Read the model definition and answer for the solid it produces. Units are mm, in the model's axes. Give positions to 0.01 mm unless a question says otherwise; leave off trailing zeros. Order: outer loops, then holes, each group sorted by start corner. A loop starts at its lowest first (then second) coordinate and runs counter-clockwise, first axis right, second up. Notation, with made-up numbers: (-25, 0.5) - (-8, 0.5) arc R27 ccw to (-8, 34.5) - close; hole circle Ø4 at (77, 1.25). An arc over 180 degrees is marked (long way). Write each question's results on one line, items separated by ' | '. Start each with the question number.
Q1. For a pull along Y with two mould halves and no side action, classify faces 1 (the face through (8, 0, 5)), 2 (the face through (14, 50.8, 5)), 3 (the face through (15.994, 28.43, 5.009)), 4 (the face through (16.365, 1.81, 5.151)) as +Y half, -Y half, draft (parallel to the pull), parting line (faces both ways), or undercut.
Q2. Find section D-D on y = 9. Give the vertices of the cut face in (x, z), and give its area (3 significant figures).
Q3. Find section A-A on z = 3.75. Give the vertices of the cut face in (x, y) (3 decimals).
Q4. Find section C-C on x = 3. Give the vertices of the cut face in (y, z).
Q5. Find section B-B on y = 2.54. Give the vertices of the cut face in (x, z), and give its area (3 significant figures).
Q6. Flat-ended cylindrical pins translate along their axes: P1, Ø3, axis at x = 4.5, z = 6, coming from the +Y side; P2, Ø2, axis at y = 44, z = 7.5, coming from the +X side. Find the tip coordinate at first contact, or state that the pin passes through.
Q7. Find the intervals of material crossed by line 1 along Y through (x, z) = (5.5, 1.25); line 2 along X through (y, z) = (26, 6); line 3 along X through (y, z) = (42.5, 1.25), in increasing order. Write a range as from..to.
from build123d import *

# Parameters (mm, degrees)
BOSS_EXTRUDE1_DEPTH     = 10.16
SKETCH2_R               = 1.905
CUT_EXTRUDE1_DEPTH      = 1
CUT_EXTRUDE1_DEPTH_BACK = 11.16


with BuildPart() as part:
    # Sketch1 → Boss-Extrude1 (new body)
    with BuildSketch(Plane.XY):
        with BuildLine():
            Line((0, 0), (16.51, 0))
            ThreePointArc((16.51, 0), (21.143005914, 25.4), (16.51, 50.8))
            Line((16.51, 50.8), (11.050639123, 50.8))
            ThreePointArc((11.050639123, 50.8), (16.008340976, 28.103171462), (12.900542854, 5.08))
            Line((12.900542854, 5.08), (0, 5.08))
            Line((0, 5.08), (0, 0))
        make_face()
    extrude(amount=BOSS_EXTRUDE1_DEPTH)

    # Sketch2 → Cut-Extrude1 (cut, two sides)
    with BuildSketch(Plane.XY.offset(10.16)) as cut_extrude1_sk:
        with Locations((14.605, 2.54)):
            Circle(SKETCH2_R)
    extrude(amount=CUT_EXTRUDE1_DEPTH, mode=Mode.SUBTRACT)
    extrude(cut_extrude1_sk.sketch, amount=-CUT_EXTRUDE1_DEPTH_BACK, mode=Mode.SUBTRACT)


solid = part.part
Working result:
1) face 1: -Y half | face 2: +Y half | face 3: undercut | face 4: undercut
2) outline: (14.02, 0) - (19.25, 0) - (19.25, 10.16) - (14.02, 10.16) - close | area: 53.1 mm²
3) outline: (0, 0) - (16.51, 0) arc R71.943 ccw to (16.51, 50.8) - (11.051, 50.8) arc R66.863 cw to (12.901, 5.08) - (0, 5.08) - close; hole circle Ø3.81 at (14.605, 2.54)
4) outline: (0, 0) - (5.08, 0) - (5.08, 10.16) - (0, 10.16) - close
5) outline: (0, 0) - (12.7, 0) - (12.7, 10.16) - (0, 10.16) - close; (16.51, 0) - (17.41, 0) - (17.41, 10.16) - (16.51, 10.16) - close | area: 138 mm²
6) P1: y = 5.08 | P2: x = 18.96
7) line 1: 0..5.08 | line 2: 16.06..21.14 | line 3: 13.84..19.08
